The model under review builds one solid part; all positions refer to its coordinate system, in mm. Face numbers are marked on the shaded views. A direction names the side the tool comes from. Round coordinates to 2 decimals unless told otherwise and drop trailing zeros. Order: outer loops, then holes, each group sorted by start corner. A loop starts at its lowest first (then second) coordinate and runs counter-clockwise, first axis right, second up.
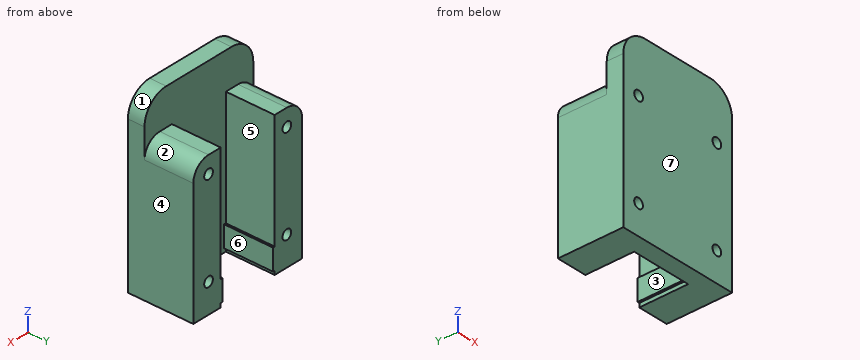
```python
from build123d import *

# Parameters (mm, degrees)
SKETCH1_W           = 30
SKETCH1_H           = 12.5
BOSS_EXTRUDE1_DEPTH = 1.6
SKETCH2_W           = 25
SKETCH2_H           = 36.5
BOSS_EXTRUDE2_DEPTH = 3.4
SKETCH3_W           = 6.3
SKETCH3_H           = 30
BOSS_EXTRUDE3_DEPTH = 10
FILLET1_R           = 5
SKETCH4_R           = 1
CUT_EXTRUDE1_DEPTH  = 16
CUT_EXTRUDE2_DEPTH  = 10
SKETCH9_W           = 0.4
SKETCH9_H           = 4.35
BOSS_EXTRUDE4_DEPTH = 10
SKETCH10_R          = 1
CUT_EXTRUDE3_DEPTH  = 16
SKETCH11_W          = 36.216016417
SKETCH11_H          = 16.907618384
CUT_EXTRUDE4_DEPTH  = 1.6


with BuildPart() as part:
    # Sketch1 → Boss-Extrude1 (new body)
    with BuildSketch(Plane(origin=(0, 0, 0), x_dir=(1, 0, 0), z_dir=(0, 1, 0))):
        with Locations((0, -6.25)):
            Rectangle(SKETCH1_W, SKETCH1_H)
    extrude(amount=BOSS_EXTRUDE1_DEPTH)

    # Sketch2 → Boss-Extrude2 (add)
    with BuildSketch(Plane(origin=(0, 1.6, 0), x_dir=(1, 0, 0), z_dir=(0, 1, 0))):
        with Locations((0, -18.25)):
            Rectangle(SKETCH2_W, SKETCH2_H)
    extrude(amount=BOSS_EXTRUDE2_DEPTH)

    # Sketch3 → Boss-Extrude3 (add)
    with BuildSketch(Plane(origin=(0, 5, 0), x_dir=(1, 0, 0), z_dir=(0, 1, 0))):
        with Locations((-9.35, -15)):
            Rectangle(SKETCH3_W, SKETCH3_H)
        with Locations((9.35, -15)):
            Rectangle(SKETCH3_W, SKETCH3_H)
    extrude(amount=BOSS_EXTRUDE3_DEPTH)

    # Fillet1
    fillet1_edges = [part.edges().sort_by_distance(p)[0] for p in [
        (12.5, 3.3, 36.5),
        (-12.5, 3.3, 36.5),
    ]]
    fillet(fillet1_edges, radius=FILLET1_R)

    # Sketch4 → Cut-Extrude1 (cut, through all)
    with BuildSketch(Plane(origin=(0, 15, 0), x_dir=(1, 0, 0), z_dir=(0, 1, 0))):
        with Locations((-9, -25.5)):
            Circle(SKETCH4_R)
        with Locations((9, -25.5)):
            Circle(SKETCH4_R)
    extrude(amount=-CUT_EXTRUDE1_DEPTH, mode=Mode.SUBTRACT)

    # Sketch5 → Cut-Extrude2 (cut)
    with BuildSketch(Plane(origin=(0, 15, 0), x_dir=(1, 0, 0), z_dir=(0, 1, 0))):
        with BuildLine():
            Line((-9, -29), (9, -29))
            ThreePointArc((9, -29), (11.474873734, -27.974873734), (12.5, -25.5))
            Line((12.5, -25.5), (17.216027855, -25.5))
            Line((17.216027855, -25.5), (17.216027855, -35.629206005))
            Line((17.216027855, -35.629206005), (-17.65496497, -35.320310993))
            Line((-17.65496497, -35.320310993), (-17.65496497, -25.5))
            Line((-17.65496497, -25.5), (-12.5, -25.5))
            ThreePointArc((-12.5, -25.5), (-11.474873734, -27.974873734), (-9, -29))
        make_face()
    extrude(amount=-CUT_EXTRUDE2_DEPTH, mode=Mode.SUBTRACT)

    # Sketch9 → Boss-Extrude4 (add)
    with BuildSketch(Plane(origin=(0, 5, 0), x_dir=(1, 0, 0), z_dir=(0, 1, 0))):
        with Locations((-6, -2.975)):
            Rectangle(SKETCH9_W, SKETCH9_H)
        with Locations((6, -2.975)):
            Rectangle(SKETCH9_W, SKETCH9_H)
    extrude(amount=BOSS_EXTRUDE4_DEPTH)

    # Sketch10 → Cut-Extrude3 (cut, through all)
    with BuildSketch(Plane(origin=(0, 15, 0), x_dir=(1, 0, 0), z_dir=(0, 1, 0))):
        with Locations((-9, -6)):
            Circle(SKETCH10_R)
        with Locations((9, -6)):
            Circle(SKETCH10_R)
    extrude(amount=-CUT_EXTRUDE3_DEPTH, mode=Mode.SUBTRACT)

    # Sketch11 → Cut-Extrude4 (cut)
    with BuildSketch(Plane.XZ):
        with Locations((-0.332022718, 6.399318006)):
            Rectangle(SKETCH11_W, SKETCH11_H)
    extrude(amount=-CUT_EXTRUDE4_DEPTH, mode=Mode.SUBTRACT)


solid = part.part
```
(1) Consider section D-D (z = 18.5). Write out the cut boundary in (x, y), and give its area (3 significant figures).
Data:
outline: (-12.5, 1.6) - (12.5, 1.6) - (12.5, 15) - (6.2, 15) - (6.2, 5) - (-6.2, 5) - (-6.2, 15) - (-12.5, 15) - close
area: 211 mm2
(2) To check wall thickness, follow probe 1 along Z at (x, y) = (9, 7.25); probe 2 along X at (y, z) = (12, 6); probe 3 along X at (y, z) = (13.5, 19). State the ranges of each line that lie inside material, in increasing order.
Data:
probe 1: z = 0 to 5, 7 to 24.5, 26.5 to 29
probe 2: x = -12.5 to -10, -8 to -6.2, 6.2 to 8, 10 to 12.5
probe 3: x = -12.5 to -6.2, 6.2 to 12.5
(3) Insertion check: pin 1 (0.8 mm diameter, centred on x = 8, y = 11, fed in from +Z). The pin has a flat end and moves straight along its axis. Give the tip position at first contact, or say it passes through.
Data:
pin 1: stops at z = 29
(4) Consider section B-B (z = 6). Write out the cut boundary in (x, y).
Data:
outline: (-12.5, 1.6) - (-10, 1.6) - (-10, 15) - (-12.5, 15) - close; (-8, 1.6) - (8, 1.6) - (8, 15) - (6.2, 15) - (6.2, 5) - (-6.2, 5) - (-6.2, 15) - (-8, 15) - close; (10, 1.6) - (12.5, 1.6) - (12.5, 15) - (10, 15) - close
(5) Draft analysis for pull direction X (two halves, no side actions). For the marked faces 4, 5, 6 and 7, state which applies: pulls with the +X half, pulls with the -X half, needs draft (parallel to the pull), parting line crosses it, or undercut.
Data:
face 4: pulls with the +X half
face 5: undercut
face 6: undercut
face 7: needs draft
(6) Consider section C-C (x = -7). Write out the cut boundary in (y, z), and give its area (3 significant figures).
Data:
outline: (1.6, 0) - (15, 0) - (15, 29) - (5, 29) - (5, 36.5) - (1.6, 36.5) - close
area: 414 mm2
(7) For the marked faces 1, 2 and 3, list the 3-axis set-ups (+Z, -Z, +X, -X, +Y, -Y) from which the entire face can be reached by the end or side of a thin tool; tool diameter is ignored.
Data:
face 1: +Z, +X, +Y, -Y
face 2: +Z, +X, +Y
face 3: +Z, -Z, +Y
(8) Consider section A-A (y = 13.25). Write out the cut boundary in (x, z).
Data:
outline: (-12.5, 0) - (-6.2, 0) - (-6.2, 0.8) - (-5.8, 0.8) - (-5.8, 5.15) - (-6.2, 5.15) - (-6.2, 29) - (-9, 29) arc R3.5 ccw to (-12.5, 25.5) - close; (5.8, 0.8) - (6.2, 0.8) - (6.2, 0) - (12.5, 0) - (12.5, 25.5) arc R3.5 ccw to (9, 29) - (6.2, 29) - (6.2, 5.15) - (5.8, 5.15) - close; hole circle Ø2 at (-9, 6); hole circle Ø2 at (-9, 25.5); hole circle Ø2 at (9, 6); hole circle Ø2 at (9, 25.5)
